Geometry check sheet. Reference: the model listing, model coordinates, mm. Face numbers are marked on the shaded views. A direction names the side the tool comes from. Give positions to 0.01 mm unless a question says otherwise; leave off trailing zeros. Loops run counter-clockwise (first coordinate to the right, second up) from the corner with the lowest first, then second, coordinate; pieces in that order, holes last. Notation, with made-up numbers: (17.25, 89.5) -> (31.25, 89.5) arc R10 cw to (31.25, 98.5) -> close; hole circle Ø2 at (-4, 26.5). An arc over 180 degrees is marked (long way). One line per item, written item: value. Start each with the question number.
(1) Tool access check on the marked faces 1, 2, 3 and 4. Record the directions out of +Z, -Z, +X, -X, +Y, -Y that give a thin tool (end or side, any length) a straight path to the whole face; none if there is none.
(2) Scan lines: line 1 along Z through (x, y) = (5.5, 60.5); line 2 along X through (y, z) = (64, 2.75); line 3 along Y through (x, z) = (3, 2.75). Record each from-to range of solid material in increasing order. Write a range as from..to.
(3) Draft check along Z on the marked faces 5, 6 and 7. Enter one of: pulls with the +Z half, pulls with the -Z half, needs draft (parallel to the pull), parting line crosses it, or undercut.
(4) Sectioned sample at D-D, the plane x = -2.25. Record the cut outline in (y, z).
(5) Gauge pin test, flat ends, axial feed: pin 1 Ø5 at (x, z) = (5, 10) entering from +Y; pin 2 Ø5 at (y, z) = (59.5, 8) entering from +X; pin 3 Ø5 at (x, z) = (8.5, 2.5) entering from +Y. Record the tip position at first contact, or that the pin passes through.
(6) Sectioned sample at A-A, the plane z = 14.75. Record the cut outline in (x, y).
(7) Sectioned sample at B-B, the plane y = 70.5. Record the cut outline in (x, z).
(8) Sectioned sample at C-C, the plane x = 0.5. Record the cut outline in (y, z), then the cut area to 3 significant figures.
from build123d import *

# Parameters (mm, degrees)
EXTRUDE_1_DEPTH     = 16
SKETCH_2_R          = 2.5
CUT_EXTRUDE_1_DEPTH = 76.727440999
SKETCH_3_W          = 10
SKETCH_3_H          = 10.5
CUT_EXTRUDE_2_DEPTH = 16
SKETCH_4_W          = 7
SKETCH_4_H          = 10
CUT_EXTRUDE_3_DEPTH = 8
FILLET_1_R          = 1.5


with BuildPart() as part:
    # 草图1 → 凸台-拉伸1 (new body)
    with BuildSketch(Plane.XY):
        with BuildLine():
            Line((-4.161479336, 67.0602), (-4.161479336, 62.0602))
            ThreePointArc((-4.161479336, 62.0602), (1.171570518, 47.59784366), (14.617205486, 40.0602))
            ThreePointArc((14.617205486, 40.0602), (8.840444726, 50.39285307), (6.838520664, 62.0602))
            Line((6.838520664, 62.0602), (6.838520664, 67.0602))
            ThreePointArc((6.838520664, 67.0602), (1.338520664, 72.5602), (-4.161479336, 67.0602))
        make_face()
    extrude(amount=EXTRUDE_1_DEPTH)

    # 草图2 → 切除-拉伸1 (cut, through all)
    with BuildSketch(Plane.XY.offset(16)):
        with Locations((1.338520664, 67.0602)):
            Circle(SKETCH_2_R)
    extrude(amount=-CUT_EXTRUDE_1_DEPTH, mode=Mode.SUBTRACT)

    # 草图3 → 切除-拉伸2 (cut)
    with BuildSketch(Plane(origin=(6.838520664, 0, 0), x_dir=(0, 0, -1), z_dir=(1, 0, 0))):
        with Locations((-8, 67.3102)):
            Rectangle(SKETCH_3_W, SKETCH_3_H)
    extrude(amount=-CUT_EXTRUDE_2_DEPTH, mode=Mode.SUBTRACT)

    # 草图4 → 切除-拉伸3 (cut)
    with BuildSketch(Plane(origin=(0, 62.0602, 0), x_dir=(1, 0, 0), z_dir=(0, 1, 0))):
        with Locations((4.838520664, -8)):
            Rectangle(SKETCH_4_W, SKETCH_4_H)
    extrude(amount=-CUT_EXTRUDE_3_DEPTH, mode=Mode.SUBTRACT)

    # 圆角1
    fillet_1_edges = [part.edges().sort_by_distance(p)[0] for p in [
        (1.338520664, 54.0602, 8),
    ]]
    fillet(fillet_1_edges, radius=FILLET_1_R)


solid = part.part
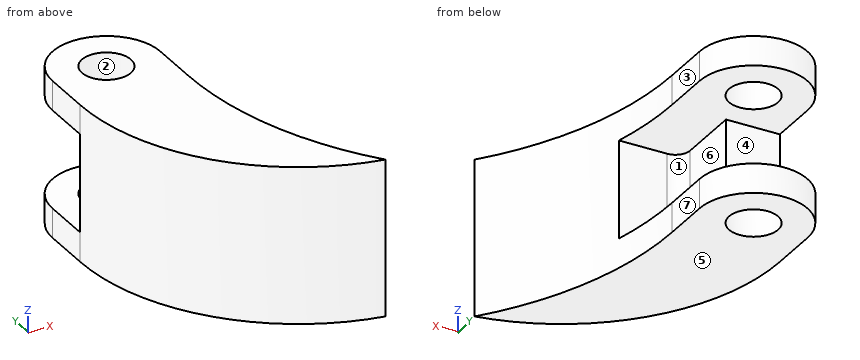
Calculated:
1. face 1: +X, +Y
1. face 2: +Z, -Z
1. face 3: +Z, -Z, +X, +Y
1. face 4: +X, -X, +Y
2. line 1: z = 0..3, 13..16
2. line 2: x = -4.16..6.84
2. line 3: y = 45.7..65.19, 68.93..72.3
3. face 5: pulls with the -Z half
3. face 6: undercut
3. face 7: needs draft
4. outline: (53.03, 0) -> (71.23, 0) -> (71.23, 3) -> (62.06, 3) -> (62.06, 13) -> (71.23, 13) -> (71.23, 16) -> (53.03, 16) -> close
5. pin 1: stops at y = 54.1
5. pin 2: stops at x = 1.34
5. pin 3: stops at y = 69.98
6. outline: (-4.16, 62.06) arc R22.28 ccw to (14.62, 40.06) arc R35 cw to (6.84, 62.06) -> (6.84, 67.06) arc R5.5 ccw to (-4.16, 67.06) -> close; hole circle Ø5 at (1.34, 67.06)
7. outline: (-2.95, 0) -> (5.63, 0) -> (5.63, 3) -> (-2.95, 3) -> close; (-2.95, 13) -> (5.63, 13) -> (5.63, 16) -> (-2.95, 16) -> close
8. outline: (48.42, 0) -> (64.71, 0) -> (64.71, 3) -> (62.06, 3) -> (62.06, 13) -> (64.71, 13) -> (64.71, 16) -> (48.42, 16) -> close; (69.42, 0) -> (72.5, 0) -> (72.5, 3) -> (69.42, 3) -> close; (69.42, 13) -> (72.5, 13) -> (72.5, 16) -> (69.42, 16) -> close
8. area: 253 mm2
